Autodesk Inventor part; units mm, degrees
ref_plane "Pracovní rovina1" through (-7.5, 0, 0) normal (1, 0, 0) x (0, 0, -1)
ref_plane "YZ Plane" through (0, 0, 0) normal (1, 0, 0) x (0, 1, 0)
ref_plane "XZ Plane" through (0, 0, 0) normal (0, 1, 0) x (-1, 0, 0)
sketch "Náčrt1" plane through (0, 0, 0) normal (0, 0, 1) x (1, 0, 0)
  line L0 (0, -3.6) -> (0, 0.6)
  line L1 (-15, 0) -> (2.5, 0)
  line L2 (-0.5196, -1) -> (-10.5144, -1)
  line L3 (0, -1.3) -> (0, -3)
  line L4 (0, -3) -> (-5.5, -3)
  line L5 (-5.5, -3) -> (-6.1348, -1.9004)
  line L6 (-6.1348, -1.9004) -> (-10.5, -1.9004)
  line L7 (-10.5, -1.9004) -> (-12.5, -0.5)
  line L8 (-12.5, -0.5) -> (-12.5, -0.2)
  line L9 (-12.5, -0.2) -> (-11.9, -0.2)
  line L10 (-11.9, -0.2) -> (-10.5144, -1)
  line L11 (-0.5196, -1) -> (0, -1.3)
  line L12 (-5.8464, -2.4) -> (-7.5, -2.4)
  line L13 (-7.5, -2.4) -> (-7.5, -1.9004)
  point P0 (0, 0)
  dimension "d0" = 6
  dimension "d1" = 0.4
  dimension "d3" = 1
  dimension "d4" = 12.5
  dimension "d5" = 10.5
  dimension "d6" = 2
  dimension "d7" = 30
  dimension "d9" = 5.5
  dimension "d10" = 120
  dimension "d36" = 0.6
  dimension "d37" = 35
  dimension "d38" = 2.6
  dimension "d39" = 30
  dimension "d40" = 4.8
  dimension "d41" = 5
revolve "Rotace1" add sketch "Náčrt1" angle 360 about axis through (-10, 0, 0) along (1, 0, 0) contours L4 L5 L6 L7 L8 L9 L10 L2 L11 L0
ref_plane "Pracovní rovina1" through (-7.5, 0, 0) normal (1, 0, 0) x (0, 0, -1)
sketch "Náčrt2" plane through (-7.5, 0, 0) normal (1, 0, 0) x (0, 0, -1)
  line L0 (0, 4.0415) -> (3.5, 2.0207)
  line L1 (3.5, 2.0207) -> (3.5, -2.0207)
  line L2 (3.5, -2.0207) -> (0, -4.0415)
  line L3 (0, -4.0415) -> (-3.5, -2.0207)
  line L4 (-3.5, -2.0207) -> (-3.5, 2.0207)
  line L5 (-3.5, 2.0207) -> (0, 4.0415)
  circle A0 centre (0, 0) radius 1.9004
  circle A1 centre (0, 0) radius 1.9004
  dimension "d13" = 7
extrude "Vysunutí1" add sketch "Náčrt2" against normal blind 3
chamfer "Zkosení1" distance 0.65 angle 45 1 edges at (0, 3, 0)
thread "Závit1"
fillet "Zaoblení1" radius 0.25 1 edges at (-10.5, 1.9004, 0)
sketch "Náčrt3" plane through (0, 0, 0) normal (0, 1, 0) x (-1, 0, 0)
  line L0 (7.5, 1.9004) -> (7.5, -1.9004)
  line L1 (7.5, 0) -> (7.5, -3.5)
  line L2 (7.5, 3.5) -> (7.5, 0)
  line L3 (7.5, 0) -> (7.5, 3.5)
  line L4 (7.5, -3.5) -> (7.5, 0)
  line L5 (10.5, 0) -> (10.5, -3.5)
  line L6 (10.5, -3.5) -> (10.5, 0)
  line L7 (10.5, 0) -> (10.5, 3.5)
  line L8 (10.5, 3.5) -> (10.5, 0)
  line L9 (10.5, -2.0306) -> (10.5, 2.0306)
  line L10 (7.5, 3.5) -> (10.5, 3.5)
  line L11 (7.5, 3.5) -> (10.5, 3.5)
  line L12 (12.6, 0) -> (-2.1, 0)
  line L13 (7.5, 3.625) -> (7.5, 4.5)
  line L14 (7.5, 4.5) -> (8.0052, 4.5)
  line L15 (8.0052, 4.5) -> (7.5, 3.625)
  line L16 (9, 3.5) -> (9, 2.759)
  line L17 (10.5, 3.625) -> (10.5, 4.5)
  line L18 (10.5, 4.5) -> (9.9948, 4.5)
  line L19 (9.9948, 4.5) -> (10.5, 3.625)
  point P0 (0, 0)
  dimension "d22" = 30
  dimension "d23" = 7.25
  dimension "d24" = 9
revolve "Rotace2" [suppressed]
sketch "Náčrt4" plane through (0, 0, 0) normal (0, 1, 0) x (-1, 0, 0)
  line L0 (7.5, 3.5) -> (10.5, 3.5)
  line L1 (9, 3.5) -> (9, 2.8)
  line L2 (9, 2.8) -> (8.8264, 2.8)
  line L3 (8.8264, 2.8) -> (8.5, 3.5)
  line L4 (9, 3.5) -> (8.5, 3.5)
  point P0 (0, 0)
  point P1 (7.7404, 3.5)
  point P2 (10.2596, 3.5)
  dimension "d26" = 25
  dimension "d27" = 1
  dimension "d28" = 0.7
revolve "Rotace3" [suppressed]
pattern_circular "Kruhové pole1" [suppressed]
revolve "Rotace4" add sketch "Náčrt1" angle 360 about axis through (-10, 0, 0) along (1, 0, 0) contours L12 L13 L6 L5
CAD build for the part. Positions are in the model's coordinates, mm. A direction names the side the tool comes from. Round coordinates to 2 decimals unless told otherwise and drop trailing zeros. Order: outer loops, then holes, each group sorted by start corner. A loop starts at its lowest first (then second) coordinate and runs counter-clockwise, first axis right, second up. Notation, with made-up numbers: (81.5, 27) - (95.5, 27) arc R14 cw to (95.5, 34) - close; hole circle Ø7 at (-6.5, -24). An arc over 180 degrees is marked (long way). Answer in a Markdown table with one row per item. Add a question column.
(1) Probe L1, parallel to Z at x = -6.5, y = 0; L2, parallel to Z at x = -4.5, y = 0. List the from-to ranges inside material, lowest first. Write a range as [from, to].
(2) Band-saw the part on C-C on y = 3.5. List the corners of the cut face in (x, z).
(3) Band-saw the part on A-A on x = -7.75. List the corners of the cut face in (y, z).
(4) Drop flat-ended pins along their axis: pin 1 Ø1 at (y, z) = (-0.5, 1.5) entering from -X; pin 2 Ø1 at (x, z) = (-3.5, -2.5) entering from +Y; pin 3 Ø2.5 at (y, z) = (0, 0) entering from +X. Give the stop position or say it passes through.
(5) Band-saw the part on D-D on x = -5.25. List the corners of the cut face in (y, z).
(6) Mould opens along Y. For faces 1 (the face through (-10.5, -2, 2)), 2 (the face through (-8.979, -3.045, 1.726)), 3 (the face through (-11.505, 0.093, 0.418)), 4 (the face through (-6, 0, -1)) say: +Y half, -Y half, draft (parallel to the pull), parting line (faces both ways), or undercut.
(7) 3-axis set-ups, long thin cutter, end or side, ignore diameter. For faces 5 (the face through (-7.5, -3, 0)), 6 (the face through (-9, 0, 3.5)), 7 (the face through (-3, 3, 0)): which of +Z, -Z, +X, -X, +Y, -Y reach the whole face in a straight line?
Data:
| question | item | result |
|---|---|---|
| 1 | L1 | z = [-2.4, -1], [1, 2.4] |
| 1 | L2 | z = [-3, -1], [1, 3] |
| 2 | outline | (-10.5, -0.94) - (-7.5, -0.94) - (-7.5, 0.94) - (-10.5, 0.94) - close |
| 3 | outline | (-4.04, 0) - (-2.02, -3.5) - (2.02, -3.5) - (4.04, 0) - (2.02, 3.5) - (-2.02, 3.5) - close; hole circle Ø2 at (0, 0) |
| 4 | pin 1 | stops at x = -11.67 |
| 4 | pin 2 | stops at y = 2.24 |
| 4 | pin 3 | stops at x = -0.09 |
| 5 | outline | circle Ø6 at (0, 0); hole circle Ø2 at (0, 0) |
| 6 | face 1 | draft |
| 6 | face 2 | -Y half |
| 6 | face 3 | undercut |
| 6 | face 4 | undercut |
| 7 | face 5 | none |
| 7 | face 6 | +Z, +X, -X, +Y, -Y |
| 7 | face 7 | +X |
